Work out the finished part from the listing and answer in its coordinate system (mm). Round coordinates to 2 decimals unless told otherwise and drop trailing zeros. Order: outer loops, then holes, each group sorted by start corner. A loop starts at its lowest first (then second) coordinate and runs counter-clockwise, first axis right, second up. Notation, with made-up numbers: (-12, 45) -> (-7, 45) arc R9 cw to (-7, 49) -> close; hole circle Ø11 at (-30.75, 14.5). An arc over 180 degrees is marked (long way). Use one line per item in the form item = value.
```python
from build123d import *

# Parameters (mm, degrees)
F1_DEPTH = 7


with BuildPart() as f1:
    # F0 (on Front) → F1 (new body)
    with BuildSketch(Plane.XZ):
        with BuildLine():
            Line((13.0394884775, 9.315168557), (16.025, 0))
            ThreePointArc((16.025, 0), (15.2603805302, 4.8909519599), (13.0394884775, 9.315168557))
        make_face()
        with BuildLine():
            ThreePointArc((13.0394884775, 9.315168557), (15.2603805302, 4.8909519599), (16.025, 0))
            ThreePointArc((16.025, 0), (15.2603805302, -4.8909519599), (13.0394884775, -9.315168557))
            Line((13.0394884775, -9.315168557), (12.1355547141, -12.1355547141))
            Line((12.1355547141, -12.1355547141), (50, 0))
            Line((50, 0), (12.1355547141, 12.1355547141))
            Line((12.1355547141, 12.1355547141), (13.0394884775, 9.315168557))
        make_face()
        with BuildLine():
            Line((11.025, 0), (16.025, 0))
            Line((16.025, 0), (13.0394884775, 9.315168557))
            ThreePointArc((13.0394884775, 9.315168557), (11.3313861685, 11.3313861685), (9.315168557, 13.0394884775))
            Line((9.315168557, 13.0394884775), (0, 16.025))
            Line((0, 16.025), (0, 11.025))
            ThreePointArc((0, 11.025), (7.7958522626, 7.7958522626), (11.025, 0))
        make_face()
        with BuildLine():
            ThreePointArc((13.0394884775, -9.315168557), (15.2603805302, -4.8909519599), (16.025, 0))
            Line((16.025, 0), (13.0394884775, -9.315168557))
        make_face()
        with BuildLine():
            Line((13.0394884775, -9.315168557), (16.025, 0))
            Line((16.025, 0), (11.025, 0))
            ThreePointArc((11.025, 0), (7.7958522626, -7.7958522626), (0, -11.025))
            Line((0, -11.025), (0, -16.025))
            Line((0, -16.025), (9.315168557, -13.0394884775))
            ThreePointArc((9.315168557, -13.0394884775), (11.3313861685, -11.3313861685), (13.0394884775, -9.315168557))
        make_face()
        with BuildLine():
            ThreePointArc((9.315168557, 13.0394884775), (11.3313861685, 11.3313861685), (13.0394884775, 9.315168557))
            Line((13.0394884775, 9.315168557), (12.1355547141, 12.1355547141))
            Line((12.1355547141, 12.1355547141), (9.315168557, 13.0394884775))
        make_face()
        with BuildLine():
            Line((12.1355547141, -12.1355547141), (13.0394884775, -9.315168557))
            ThreePointArc((13.0394884775, -9.315168557), (11.3313861685, -11.3313861685), (9.315168557, -13.0394884775))
            Line((9.315168557, -13.0394884775), (12.1355547141, -12.1355547141))
        make_face()
        with BuildLine():
            Line((0, 16.025), (9.315168557, 13.0394884775))
            ThreePointArc((9.315168557, 13.0394884775), (4.8909519599, 15.2603805302), (0, 16.025))
        make_face()
        with BuildLine():
            ThreePointArc((0, 16.025), (4.8909519599, 15.2603805302), (9.315168557, 13.0394884775))
            Line((9.315168557, 13.0394884775), (12.1355547141, 12.1355547141))
            Line((12.1355547141, 12.1355547141), (0, 50))
            Line((0, 50), (-12.1347763783, 12.1379832191))
            Line((-12.1347763783, 12.1379832191), (-9.3109210563, 13.0425217686))
            ThreePointArc((-9.3109210563, 13.0425217686), (-4.8884667156, 15.2611768278), (0, 16.025))
        make_face()
        with BuildLine():
            Line((12.1355547141, -12.1355547141), (9.315168557, -13.0394884775))
            ThreePointArc((9.315168557, -13.0394884775), (4.8909519599, -15.2603805302), (0, -16.025))
            ThreePointArc((0, -16.025), (-4.8884667156, -15.2611768278), (-9.3109210563, -13.0425217686))
            Line((-9.3109210563, -13.0425217686), (-12.1347763783, -12.1379832191))
            Line((-12.1347763783, -12.1379832191), (0, -50))
            Line((0, -50), (12.1355547141, -12.1355547141))
        make_face()
        with BuildLine():
            ThreePointArc((0, -16.025), (4.8909519599, -15.2603805302), (9.315168557, -13.0394884775))
            Line((9.315168557, -13.0394884775), (0, -16.025))
        make_face()
        with BuildLine():
            ThreePointArc((0, -11.025), (-11.025, 0), (0, 11.025))
            Line((0, 11.025), (0, 16.025))
            Line((0, 16.025), (-9.3109210563, 13.0425217686))
            ThreePointArc((-9.3109210563, 13.0425217686), (-11.3295406823, 11.3332313542), (-13.0394884775, 9.315168557))
            Line((-13.0394884775, 9.315168557), (-16.025, 0))
            Line((-16.025, 0), (-13.0394884775, -9.315168557))
            ThreePointArc((-13.0394884775, -9.315168557), (-11.3295406823, -11.3332313542), (-9.3109210563, -13.0425217686))
            Line((-9.3109210563, -13.0425217686), (0, -16.025))
            Line((0, -16.025), (0, -11.025))
        make_face()
        with BuildLine():
            Line((-9.3109210563, 13.0425217686), (0, 16.025))
            ThreePointArc((0, 16.025), (-4.8884667156, 15.2611768278), (-9.3109210563, 13.0425217686))
        make_face()
        with BuildLine():
            ThreePointArc((-9.3109210563, -13.0425217686), (-4.8884667156, -15.2611768278), (0, -16.025))
            Line((0, -16.025), (-9.3109210563, -13.0425217686))
        make_face()
        with BuildLine():
            ThreePointArc((-13.0394884775, 9.315168557), (-11.3295406823, 11.3332313542), (-9.3109210563, 13.0425217686))
            Line((-9.3109210563, 13.0425217686), (-12.1347763783, 12.1379832191))
            Line((-12.1347763783, 12.1379832191), (-13.0394884775, 9.315168557))
        make_face()
        with BuildLine():
            Line((-13.0394884775, 9.315168557), (-12.1347763783, 12.1379832191))
            Line((-12.1347763783, 12.1379832191), (-50.0280298293, 0))
            Line((-50.0280298293, 0), (-12.1347763783, -12.1379832191))
            Line((-12.1347763783, -12.1379832191), (-13.0394884775, -9.315168557))
            ThreePointArc((-13.0394884775, -9.315168557), (-15.2603805302, -4.8909519599), (-16.025, 0))
            ThreePointArc((-16.025, 0), (-15.2603805302, 4.8909519599), (-13.0394884775, 9.315168557))
        make_face()
        with BuildLine():
            Line((-12.1347763783, -12.1379832191), (-9.3109210563, -13.0425217686))
            ThreePointArc((-9.3109210563, -13.0425217686), (-11.3295406823, -11.3332313542), (-13.0394884775, -9.315168557))
            Line((-13.0394884775, -9.315168557), (-12.1347763783, -12.1379832191))
        make_face()
        with BuildLine():
            Line((-16.025, 0), (-13.0394884775, 9.315168557))
            ThreePointArc((-13.0394884775, 9.315168557), (-15.2603805302, 4.8909519599), (-16.025, 0))
        make_face()
        with BuildLine():
            ThreePointArc((-16.025, 0), (-15.2603805302, -4.8909519599), (-13.0394884775, -9.315168557))
            Line((-13.0394884775, -9.315168557), (-16.025, 0))
        make_face()
    extrude(amount=F1_DEPTH)


solid = f1.part
```
Item 1: Consider line 1 along X through (y, z) = (-1.75, -43.5); line 2 along Z through (x, y) = (-16, -6.5); line 3 along Z through (x, y) = (41, -6). Determine where each line is inside the solid, lowest interval first.
Findings:
line_1 = -2.08 to 2.08
line_2 = -10.9 to 10.9
line_3 = -2.88 to 2.88
Item 2: The part is cut by section B-B, the plane x = 9. Give the vertices of the cut face in (y, z).
Findings:
outline = (-7, -21.92) -> (0, -21.92) -> (0, -6.37) -> (-7, -6.37) -> close; (-7, 6.37) -> (0, 6.37) -> (0, 21.92) -> (-7, 21.92) -> close
Item 3: The part is cut by section C-C, the plane z = -24. Give the vertices of the cut face in (x, y), and give its area (3 significant figures).
Findings:
outline = (-8.33, -7) -> (8.33, -7) -> (8.33, 0) -> (-8.33, 0) -> close
area = 117 mm^2
Item 4: The part is cut by section A-A, the plane y = -3. Give the vertices of the cut face in (x, z) (3 decimals).
Findings:
outline = (-50.028, 0) -> (-12.135, -12.138) -> (0, -50) -> (12.136, -12.136) -> (50, 0) -> (12.136, 12.136) -> (0, 50) -> (-12.135, 12.138) -> close; hole circle Ø22.05 at (0, 0)
Item 5: The part is cut by section D-D, the plane x = -30. Give the vertices of the cut face in (y, z).
Findings:
outline = (-7, -6.42) -> (0, -6.42) -> (0, 6.42) -> (-7, 6.42) -> close
